from build123d import *

# Parameters (mm, degrees)
F1_DEPTH = 10


with BuildPart() as f1:
    # F0 (on Front) → F1 (new body)
    with BuildSketch(Plane.XZ):
        with BuildLine():
            Line((-2.5, -40), (15, -40))
            Line((15, -40), (15, -29))
            Line((15, -29), (5.5, -29))
            ThreePointArc((5.5, -29), (3.156854, -34.656854), (-2.5, -37))
            Line((-2.5, -37), (-2.5, -40))
        make_face()
        with BuildLine():
            ThreePointArc((-14.909674, -29), (-10.791562, -36.854143), (-2.5, -40))
            Line((-2.5, -40), (-2.5, -37))
            ThreePointArc((-2.5, -37), (-8.156854, -34.656854), (-10.5, -29))
            Line((-10.5, -29), (-14.909674, -29))
        make_face()
        with BuildLine():
            Line((5.5, -29), (15, -29))
            Line((15, -29), (15, 29))
            Line((15, 29), (5.5, 29))
            ThreePointArc((5.5, 29), (3.156854, 23.343146), (-2.5, 21))
            Line((-2.5, 21), (-2.5, -21))
            ThreePointArc((-2.5, -21), (3.156854, -23.343146), (5.5, -29))
        make_face()
        with BuildLine():
            ThreePointArc((-15, -27.5), (-14.977398, -28.251359), (-14.909674, -29))
            Line((-14.909674, -29), (-10.5, -29))
            ThreePointArc((-10.5, -29), (-8.156854, -23.343146), (-2.5, -21))
            Line((-2.5, -21), (-2.5, 21))
            ThreePointArc((-2.5, 21), (-8.156854, 23.343146), (-10.5, 29))
            Line((-10.5, 29), (-14.909674, 29))
            ThreePointArc((-14.909674, 29), (-14.977398, 28.251359), (-15, 27.5))
            Line((-15, 27.5), (-15, -27.5))
        make_face()
        with BuildLine():
            Line((5.5, 29), (15, 29))
            Line((15, 29), (15, 40))
            Line((15, 40), (-2.5, 40))
            Line((-2.5, 40), (-2.5, 37))
            ThreePointArc((-2.5, 37), (3.156854, 34.656854), (5.5, 29))
        make_face()
        with BuildLine():
            Line((-2.5, 37), (-2.5, 40))
            ThreePointArc((-2.5, 40), (-10.791562, 36.854143), (-14.909674, 29))
            Line((-14.909674, 29), (-10.5, 29))
            ThreePointArc((-10.5, 29), (-8.156854, 34.656854), (-2.5, 37))
        make_face()
    extrude(amount=F1_DEPTH)


solid = f1.part
Work out the finished part from the listing and answer in its coordinate system (mm). Coordinates: 2 decimals unless noted, no trailing zeros. Write each loop counter-clockwise with the first axis right and the second up, starting at its lowest first coordinate (ties: lowest second). Pieces come first, ordered by that corner, then holes. Notation, with made-up numbers: M -5.5,-37 L 26.5,-37 A17 ccw 26.5,-9 Z; hole C 38.25,30 d4. An arc over 180 degrees is marked long. Answer as CSV lines item,"result". Start each with the question number.
Item 1: Section B-B on x = -6.5 is taken. Write down the section's boundary in (y, z), and give its area (3 significant figures).
Item 2: Section A-A on y = -5 is taken. Write down the section's boundary in (x, z).
Item 3: Consider L1, parallel to Z at x = -2.5, y = -0.5; L2, parallel to Z at x = -8, y = -6.5; L3, parallel to X at y = -2.75, z = 33.5. Determine where each line is inside the solid, lowest interval first.
Item 4: Section C-C on x = -1.25 is taken. Write down the section's boundary in (y, z), and give its area (3 significant figures).
Checks:
1,outline,"M -10,-39.34 L 0,-39.34 L 0,-35.93 L -10,-35.93 Z; M -10,-22.07 L 0,-22.07 L 0,22.07 L -10,22.07 Z; M -10,35.93 L 0,35.93 L 0,39.34 L -10,39.34 Z"
1,area,"510 mm²"
2,outline,"M -15,-27.5 A12.5 ccw -14.91,-29 A12.5 ccw -2.5,-40 L 15,-40 L 15,40 L -2.5,40 A12.5 ccw -14.91,29 A12.5 ccw -15,27.5 Z; hole M -10.5,-29 A8 ccw -2.5,-37 A8 ccw 5.5,-29 A8 ccw -2.5,-21 A8 ccw Z; hole M -10.5,29 A8 ccw -2.5,21 A8 ccw 5.5,29 A8 ccw -2.5,37 A8 ccw Z"
3,L1,"z = -40 to -37, -21 to 21, 37 to 40"
3,L2,"z = -38.72 to -34.81, -23.19 to 23.19, 34.81 to 38.72"
3,L3,"x = -13.47 to -9.11, 4.11 to 15"
4,outline,"M -10,-40 L 0,-40 L 0,-36.9 L -10,-36.9 Z; M -10,-21.1 L 0,-21.1 L 0,21.1 L -10,21.1 Z; M -10,36.9 L 0,36.9 L 0,40 L -10,40 Z"
4,area,"484 mm²"
